Model file for the job. Use its own axes, mm. Give positions to 0.01 mm unless a question says otherwise; leave off trailing zeros. Loops run counter-clockwise (first coordinate to the right, second up) from the corner with the lowest first, then second, coordinate; pieces in that order, holes last. Notation, with made-up numbers: (-19, -34.75) -> (-4, -34.75) arc R37 ccw to (-4, 4.25) -> close; hole circle Ø8 at (49.5, 79.25). An arc over 180 degrees is marked (long way). Use CSV: the item, a comma, the result in double quotes. Start each with the question number.
(1) Cut at D-D on x = 0. Write the cut outline in (y, z), then the cut area to 3 significant figures.
(2) Cut at A-A on x = 1.75. Write the cut outline in (y, z), then the cut area to 3 significant figures.
(3) Drill centre lines: probe 1 along Z at (x, y) = (1.75, 0.1); probe 2 along Z at (x, y) = (2, 0.1); probe 3 along X at (y, z) = (0.05, -1). Where is each one in solid material? Low to high.
(4) Cut at B-B on y = 0.2. Write the cut outline in (x, z), then the cut area to 3 significant figures.
(5) Cut at C-C on z = 0.25. Write the cut outline in (x, y), then the cut area to 3 significant figures.
from build123d import *

# Parameters (mm, degrees)
BOSS_EXTRUDE1_DEPTH = 0.254


with BuildPart() as part:
    # Sketch1 → Boss-Extrude1 (new body)
    with BuildSketch(Plane(origin=(0, 0, 0), x_dir=(1, 0, 0), z_dir=(0, 1, 0))):
        with BuildLine():
            Line((-0.990450861, 2.338932896), (-0.990450861, 4.98251012))
            ThreePointArc((-0.990450861, 4.98251012), (-5.08, 0), (-0.990450861, -4.98251012))
            Line((-0.990450861, -4.98251012), (-0.990450861, -2.338932896))
            ThreePointArc((-0.990450861, -2.338932896), (-2.54, 0), (-0.990450861, 2.338932896))
        make_face()
        with BuildLine():
            ThreePointArc((0.990450861, 4.98251012), (0, 5.08), (-0.990450861, 4.98251012))
            Line((-0.990450861, 4.98251012), (-0.990450861, 2.338932896))
            ThreePointArc((-0.990450861, 2.338932896), (0, 2.54), (0.990450861, 2.338932896))
            Line((0.990450861, 2.338932896), (0.990450861, 4.98251012))
        make_face()
        with BuildLine():
            ThreePointArc((5.08, 0), (3.926696472, 3.222957464), (0.990450861, 4.98251012))
            Line((0.990450861, 4.98251012), (0.990450861, 2.338932896))
            ThreePointArc((0.990450861, 2.338932896), (2.11746844, 1.40282836), (2.54, 0))
            ThreePointArc((2.54, 0), (2.11746844, -1.40282836), (0.990450861, -2.338932896))
            Line((0.990450861, -2.338932896), (0.990450861, -4.98251012))
            ThreePointArc((0.990450861, -4.98251012), (3.926696472, -3.222957464), (5.08, 0))
        make_face()
    extrude(amount=BOSS_EXTRUDE1_DEPTH)


solid = part.part
Check result:
1,outline,"(0, -5.08) -> (0.25, -5.08) -> (0.25, -2.54) -> (0, -2.54) -> close"
1,area,"0.645 mm²"
2,outline,"(0, -4.77) -> (0.25, -4.77) -> (0.25, -1.84) -> (0, -1.84) -> close; (0, 1.84) -> (0.25, 1.84) -> (0.25, 4.77) -> (0, 4.77) -> close"
2,area,"1.49 mm²"
3,probe 1,"-4.77 to -1.84, 1.84 to 4.77"
3,probe 2,"-4.67 to -1.57, 1.57 to 4.67"
3,probe 3,"-4.98 to -2.33, 2.33 to 4.98"
4,outline,"(-0.99, 2.34) -> (-0.99, 4.98) arc R5.08 ccw (long way) to (0.99, 4.98) -> (0.99, 2.34) arc R2.54 cw (long way) to start"
4,area,"55.7 mm²"
5,outline,"(-5.07, 0) -> (-2.53, 0) -> (-2.53, 0.25) -> (-5.07, 0.25) -> close; (2.53, 0) -> (5.07, 0) -> (5.07, 0.25) -> (2.53, 0.25) -> close"
5,area,"1.29 mm²"
